Drawing for the job (mm, zero at the part's lowest x, y, z). Round coordinates to 2 decimals unless told otherwise and drop trailing zeros. Order: outer loops, then holes, each group sorted by start corner. A loop starts at its lowest first (then second) coordinate and runs counter-clockwise, first axis right, second up. Notation, with made-up numbers: (-6.75, 56.25) - (31.25, 56.25) arc R8 cw to (31.25, 67.25) - close; hole circle Ø1 at (-27.5, 5.5). An arc over 180 degrees is marked (long way). Put each result on its own line as item: value. Start each with the question number.
Item 1: Saw through at A-A on z = 10. List the corners of the cut face in (x, y).
Item 2: Probe probe 1 along Z at (x, y) = (30, 1.45); probe 2 along Z at (x, y) = (31, 0.75); probe 3 along Z at (x, y) = (38, 3.45). List the from-to ranges inside material, lowest first.
Item 3: Saw through at D-D on z = 30. List the corners of the cut face in (x, y).
Item 4: Saw through at B-B on y = 0.95. List the corners of the cut face in (x, z), plus the area to 3 significant figures.
Item 5: Pin check, flat tip, straight feed: pin 1 Ø2 at (x, z) = (35.5, 16) entering from -Y. Stop position of the tip, or through.
Item 6: Saw through at C-C on x = 30. List the corners of the cut face in (y, z).
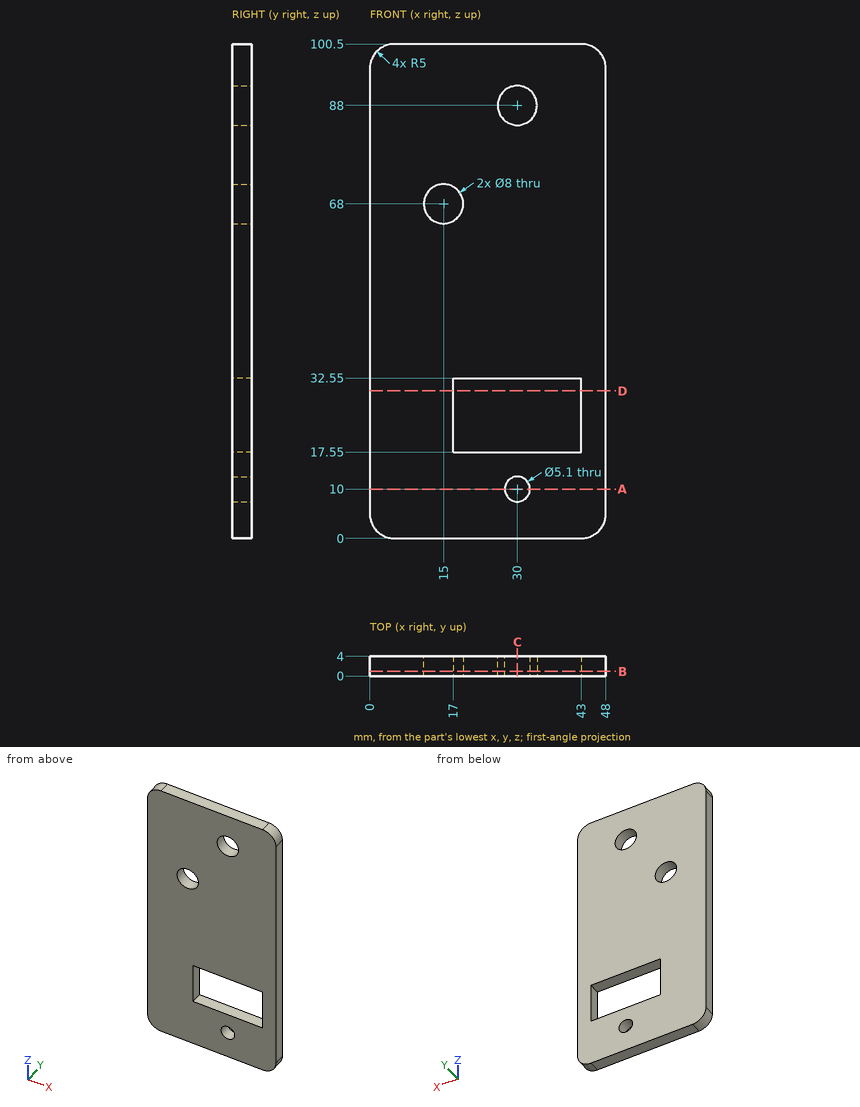
Results found:
1. outline: (0, 0) - (27.45, 0) - (27.45, 4) - (0, 4) - close; (32.55, 0) - (48, 0) - (48, 4) - (32.55, 4) - close
2. probe 1: z = 0 to 7.45, 12.55 to 17.55, 32.55 to 84, 92 to 100.5
2. probe 2: z = 0 to 7.65, 12.35 to 17.55, 32.55 to 84.13, 91.87 to 100.5
2. probe 3: z = 0 to 17.55, 32.55 to 100.5
3. outline: (0, 0) - (17, 0) - (17, 4) - (0, 4) - close; (43, 0) - (48, 0) - (48, 4) - (43, 4) - close
4. outline: (0, 5) arc R5 ccw to (5, 0) - (43, 0) arc R5 ccw to (48, 5) - (48, 95.5) arc R5 ccw to (43, 100.5) - (5, 100.5) arc R5 ccw to (0, 95.5) - close; hole circle Ø8 at (15, 68); hole (17, 17.55) - (43, 17.55) - (43, 32.55) - (17, 32.55) - close; hole circle Ø8 at (30, 88); hole circle Ø5.1 at (30, 10)
4. area: 4,290 mm²
5. pin 1: stops at y = 0
6. outline: (0, 0) - (4, 0) - (4, 7.45) - (0, 7.45) - close; (0, 12.55) - (4, 12.55) - (4, 17.55) - (0, 17.55) - close; (0, 32.55) - (4, 32.55) - (4, 84) - (0, 84) - close; (0, 92) - (4, 92) - (4, 100.5) - (0, 100.5) - close
